```python
from build123d import *
from OCP.BRepFilletAPI import BRepFilletAPI_MakeChamfer

# Parameters (mm, degrees)
CHAMFER1_SIZE  = 3
CHAMFER1_SIZE2 = 3.300188603
CHAMFER2_SIZE  = 0.5


with BuildPart() as part:
    # Sketch1 → Revolve1 (revolve)
    with BuildSketch(Plane(origin=(0, 0, 0), x_dir=(1, 0, 0), z_dir=(0, 1, 0))):
        Polygon((0, 0), (0, 12.5), (16.5, 12.5), (19.780824882, 50), (180.219175118, 50), (183.5, 12.5), (200, 12.5), (200, 0), align=None)
    revolve(axis=Axis((200, 0, 0), (-1, 0, 0)))

    # Chamfer1: one chamfer whose edges measure the first distance from different faces: ONE call of the kernel's chamfer builder (chamfer() names one face for all edges)
    chamfer1_edges_1 = [part.edges().sort_by_distance(p)[0] for p in [
        (180.219175118, 0, 50),
    ]]
    chamfer1_side_1 = [part.faces().sort_by_distance(p)[0] for p in [
        (100, 0, 50),
    ]]
    chamfer1_edges_2 = [part.edges().sort_by_distance(p)[0] for p in [
        (19.780824882, 0, 50),
    ]]
    chamfer1_side_2 = [part.faces().sort_by_distance(p)[0] for p in [
        (18.140412441, 0, 31.25),
    ]]
    chamfer1 = BRepFilletAPI_MakeChamfer(part.part.solid().wrapped)
    for e in chamfer1_edges_1:
        chamfer1.Add(CHAMFER1_SIZE, CHAMFER1_SIZE2, e.wrapped, chamfer1_side_1[0].wrapped)  # the first distance lies on this face
    for e in chamfer1_edges_2:
        chamfer1.Add(CHAMFER1_SIZE, CHAMFER1_SIZE2, e.wrapped, chamfer1_side_2[0].wrapped)  # the first distance lies on this face
    add(Compound.cast(chamfer1.Shape()), mode=Mode.REPLACE)

    # Chamfer2
    chamfer2_edges = [part.edges().sort_by_distance(p)[0] for p in [
        (200, 0, 12.5),
        (0, 0, 12.5),
    ]]
    chamfer(chamfer2_edges, length=CHAMFER2_SIZE)

    # Sketch3 → M10 Clearance Hole1 (revolve, cut)
    with BuildSketch(Plane(origin=(200, 0, 0), x_dir=(0, 0, -1), z_dir=(0, 1, 0))):
        Polygon((0, 0), (0, 59), (5.5, 55.695266595), (5.5, 0.025), (5.525, 0), align=None)
    m10_clearance_hole1 = revolve(axis=Axis((206.35, 0, 0), (-1, 0, 0)), mode=Mode.SUBTRACT)

    # Mirror1: M10 Clearance Hole1 across plane
    add(m10_clearance_hole1.mirror(Plane(origin=(100, 0, 0), x_dir=(0, 0, 1), z_dir=(1, 0, 0))), mode=Mode.SUBTRACT)


solid = part.part
```
Input: part model. Units: mm. Frame: model coordinates. A direction names the side the tool comes from. Coordinates: 2 decimals unless noted, no trailing zeros. Loops run counter-clockwise (first coordinate to the right, second up) from the corner with the lowest first, then second, coordinate; pieces in that order, holes last. Notation, with made-up numbers: M -37.5,-31.75 L 15.5,-31.75 A36 ccw 15.5,5.25 Z; hole C 7,6.25 d8. An arc over 180 degrees is marked long. Answer in a Markdown table with one row per item.
1. Material intervals for line 1 (Y direction, x = 161.5, z = 0); line 2 (Y direction, x = 16, z = 0), sorted ascending.
Response:
| item | result |
|---|---|
| line 1 | y = -50 to -5.5, 5.5 to 50 |
| line 2 | y = -12.5 to -5.5, 5.5 to 12.5 |
2. Reachability of faces 4 (the cylindrical face through (191.612, -3.755, -11.923)), 5 (the cylindrical face through (27.47, 5.37, 1.19)), 6 (the cylindrical face through (101.23, 44.36, -23.07)) from +Z, -Z, +X, -X, +Y, -Y: full face, straight path, thin tool, end or side. Return the list, or none.
Response:
| item | result |
|---|---|
| face 4 | +X |
| face 5 | -X |
| face 6 | +X, -X |
3. Section A-A, the plane x = 173. Output: boundary loops of the cut face in (y, z).
Response:
| item | result |
|---|---|
| outline | C 0,0 d100; hole C 0,0 d11 |
4. First-contact query: pin 1 (3 mm diameter, centred on x = 165, y = 31.5, fed in from +Z); pin 2 (3 mm diameter, centred on y = -6, z = -34.5, fed in from -X); pin 3 (4 mm diameter, centred on x = 72, z = -39, fed in from +Y). Flat tips, straight axial feed; report the tip coordinate or a pass-through.
Response:
| item | result |
|---|---|
| pin 1 | stops at z = 40 |
| pin 2 | stops at x = 18.34 |
| pin 3 | stops at y = 33.63 |
5. Section B-B, the plane x = 138.5. Output: boundary loops of the cut face in (y, z), then the cut area to 3 significant figures.
Response:
| item | result |
|---|---|
| outline | C 0,0 d100 |
| area | 7,850 mm2 |
6. Draft query along Y for faces 1 (the flat face through (200, 2.5, -5.2)), 2 (the conical face through (141.574, 0.932, 0.207)), 3 (the conical face through (183.355, 13.824, 3.07)). Return one class per face: pulls with the +Y half, pulls with the -Y half, needs draft (parallel to the pull), parting line crosses it, or undercut.
Response:
| item | result |
|---|---|
| face 1 | needs draft |
| face 2 | undercut |
| face 3 | parting line crosses it |
